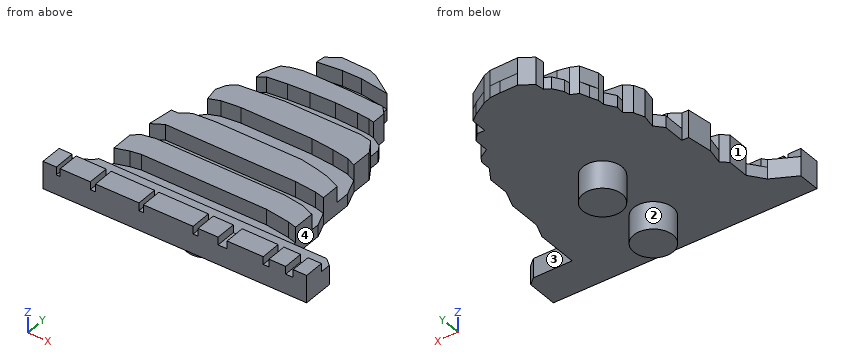
from build123d import *

# Parameters (mm, degrees)
F2_DEPTH  = 0.762
F4_DEPTH  = 1.016
F6_DEPTH  = 1.016
F8_DEPTH  = 0.5258
F0_R      = 12.7
F10_DEPTH = 0.50448
F11_R     = 1.2664455111
F11_R_2   = 1.2714517288
F12_DEPTH = 1.778


with BuildPart() as f2:
    # F1 (on face) → F2 (new body)
    with BuildSketch(Plane.XY):
        Polygon((-8.301156573, -6.202286575), (-8.301156573, -7.6132696122), (8.7365023792, -7.5040537175), (8.7365023792, -5.5138876204), (8.2679493353, -5.1142387092), (5.7544014417, -5.1142387092), (5.7544014417, -2.8919042088), (5.7544014417, -2.4577556178), (5.3745214827, -1.4809214044), (5.3745214827, -0.9925042978), (5.3745214827, 0), (5.3745214827, 0.6355526857), (4.9403728917, 1.7751924461), (4.9403728917, 2.4806838483), (4.9403728917, 3.1319067348), (4.3976870365, 4.000203684), (4.3976870365, 4.6514268033), (4.1806129739, 5.0313062966), (3.529390553, 5.4111862555), (3.529390553, 6.3337520696), (3.0952417292, 6.8221688271), (2.6068247389, 6.8221688271), (2.6068247389, 7.853272371), (2.1184075158, 8.2331513986), (1.1958420509, 8.7758377194), (0.6879131543, 8.9615155011), (0, 9.0042492375), (-1.1481875752, 9.0042492375), (-1.9346952904, 8.4792003036), (-2.0060034003, 7.9075405374), (-2.3858833592, 7.6904660091), (-2.7657633182, 7.0935124531), (-2.8200319503, 6.7136320285), (-3.3084489405, 6.4965579659), (-3.5255230032, 5.8996034786), (-3.7425975315, 5.4111862555), (-3.7425975315, 4.9770376645), (-4.1767461225, 4.3258150108), (-4.1224774905, 3.8373982534), (-4.5566260815, 3.4575182945), (-4.8279687762, 2.8062951751), (-4.6651633456, 1.9379982259), (-5.1535801031, 1.3953124871), (-5.1535801031, 0), (-5.5877286941, 0), (-5.8048027568, -1.6437270679), (-5.5877286941, -2.6748299133), (-6.0218772851, -3.0547098722), (-6.0218772851, -4.4656926766), (-6.7273690365, -5.3882584907), align=None)
    extrude(amount=F2_DEPTH)

    # F3 (on face) → F4 (join)
    with BuildSketch(Plane.XY.offset(0.762)):
        Polygon((-8.301156573, -7.6132696122), (8.7365023792, -7.5040537175), (8.7365023792, -5.5138876204), (8.2679493353, -5.1142387092), (5.7544014417, -5.1142387092), (-6.5178244245, -5.1142387092), (-6.7273690365, -5.3882584907), (-8.301156573, -6.202286575), align=None)
    extrude(amount=F4_DEPTH)

    # F5 (on face) → F6 (join)
    with BuildSketch(Plane.XY.offset(0.762)):
        Polygon((-1.9346952904, 8.4792003036), (-2.0060034003, 7.9075405374), (-0.4768302024, 8.0958995968), (0.7676923415, 8.1118550152), (2.6068247389, 7.853272371), (1.1958420509, 8.7758377194), (0.6879131543, 8.9615155011), (-1.1481875752, 9.0042492375), align=None)
        Polygon((-2.1202382632, 6.8673328497), (-2.8200319503, 6.7136320285), (-3.3084489405, 6.4965579659), (-3.7425975315, 5.4111862555), (-3.7425975315, 4.9770376645), (-3.3328498248, 5.2877464332), (-2.0883274265, 5.4473006167), (-0.7002060302, 5.5430331267), (0.927246525, 5.6068548001), (2.3791892454, 5.5589885451), (3.1769601628, 5.4951668717), (3.529390553, 5.4111862555), (3.529390553, 6.3337520696), (3.0952417292, 6.8221688271), (2.6068247389, 6.8221688271), (0.9432018269, 6.8992436863), (-1.290556509, 6.8992436863), align=None)
        Polygon((-2.7597796666, 3.9888094114), (-4.1224774905, 3.8373982534), (-4.5566260815, 3.4575182945), (-4.8279687762, 2.8062951751), (-4.6651633456, 1.9379982259), (-4.0006320924, 2.1927114576), (-2.8066006489, 2.334858058), (-1.3140613446, 2.334858058), (0.1642632997, 2.334858058), (1.7989494372, 2.334858058), (3.263059305, 2.2069262341), (4.3575884774, 2.0363503136), (4.9403728917, 1.7751924461), (4.9403728917, 3.1319067348), (4.3976870365, 4.000203684), (3.6326404661, 4.1401199996), (2.3959649261, 4.1401199996), (0.8465670398, 4.1401199996), (-1.2998466846, 4.1401199996), align=None)
        Polygon((-5.5877286941, 0), (-5.8048027568, -1.6437270679), (-5.076691974, -1.2083072215), (-3.9773182943, -1.2083072215), (-1.5074934345, -1.2083072215), (0.9020918515, -1.2083072215), (3.3719167113, -1.2083072215), (4.7423685901, -1.3287864858), (5.3745214827, -1.4809214044), (5.3745214827, -0.2745929523), (4.4110501185, 0.1470844581), (3.5074558109, 0.3579231852), (2.4683221709, 0.5386420526), (0, 0.5386420526), (-3.1490232795, 0.5386420526), (-4.53453511, 0.4181628174), (-5.1535801031, 0), align=None)
        Polygon((-5.5877286941, -2.6748299133), (-6.0218772851, -3.0547098722), (-6.0218772851, -4.4656926766), (-5.1821111701, -4.1901692748), (-4.5194751583, -4.0696901269), (-2.0044704434, -4.0696901269), (1.4593084343, -4.0696901269), (3.5978152882, -4.0696901269), (5.1791053265, -4.2805285193), (5.7544014417, -4.4461875223), (5.7544014417, -3.0154963024), (4.9230875447, -2.6841785293), (3.5978152882, -2.4995030768), (1.3388292864, -2.4995030768), (-2.4412076455, -2.4995030768), (-4.7549253743, -2.4995030768), align=None)
    extrude(amount=F6_DEPTH)

    # F7 (on face) → F8 (cut)
    with BuildSketch(Plane.XY.offset(1.778)):
        Polygon((-6.7273690365, -5.3882584907), (-8.301156573, -6.202286575), (8.7365023792, -6.202286575), (8.7365023792, -5.5138876204), (8.2679493353, -5.1142387092), (-6.5178244245, -5.1142387092), align=None)
    extrude(amount=-F8_DEPTH, mode=Mode.SUBTRACT)

    # F9 (on face) + F0 (on Top) → F10 (cut)
    with BuildSketch(Plane.XY.offset(1.778)):
        Polygon((-7.4496113843, -6.202286575), (-7.4406019717, -7.6077532299), (-7.1891224943, -7.60614118), (-7.1891224943, -6.202286575), align=None)
        Polygon((-5.2457139827, -6.202286575), (-5.2457139827, -7.593683418), (-4.905404364, -7.5915019435), (-4.9143096015, -6.202286575), align=None)
        Polygon((-2.0974383224, -6.202286575), (-2.0974383224, -7.5735021394), (-1.8112884347, -7.571667843), (-1.8200665304, -6.202286575), align=None)
        Polygon((7.377400318, -6.202286575), (7.3858004916, -7.5127120734), (7.8655239195, -7.5096369195), (7.8655239195, -6.202286575), align=None)
        Polygon((5.9232353463, -6.202286575), (5.9316952713, -7.522033272), (6.3001448289, -7.519671413), (6.3001448289, -6.202286575), align=None)
        Polygon((3.014677437, -6.202286575), (3.014677437, -7.5407321269), (3.5971800525, -7.5369981313), (3.5886241988, -6.202286575), align=None)
        Polygon((1.3927921775, -6.202286575), (1.4014382575, -7.5510734162), (1.7183985864, -7.5490416168), (1.7097655308, -6.202286575), align=None)
    with BuildSketch(Plane.XY):
        Circle(F0_R)
    extrude(amount=-F10_DEPTH, mode=Mode.SUBTRACT)

    # F11 (on face) → F12 (join)
    with BuildSketch(Plane.XY):
        Circle(F11_R)
        with Locations((0, -4.4713900425)):
            Circle(F11_R_2)
    extrude(amount=-F12_DEPTH)


solid = f2.part
The model under review builds one solid part; all positions refer to its coordinate system, in mm. Face numbers are marked on the shaded views. A direction names the side the tool comes from. Round coordinates to 2 decimals unless told otherwise and drop trailing zeros. Order: outer loops, then holes, each group sorted by start corner. A loop starts at its lowest first (then second) coordinate and runs counter-clockwise, first axis right, second up. Notation, with made-up numbers: (48.5, 75.5) -> (81.5, 75.5) arc R10 cw to (81.5, 93.5) -> close; hole circle Ø11 at (-17, -22.5). An arc over 180 degrees is marked (long way). Use CSV: the item, a comma, the result in double quotes. Start each with the question number.
(1) Insertion check: pin 1 (0.5 mm diameter, centred on y = -4, z = 1, fed in from +X); pin 2 (1.5 mm diameter, centred on x = -0.5, y = 6, fed in from -Z); pin 3 (1.5 mm diameter, centred on x = -4, z = -1.5, fed in from +Y); pin 4 (1.5 mm diameter, centred on y = 7, z = 0, fed in from +X). Each pin has a flat end and moves straight along its axis. Give the tip position at first contact, or say it passes through.
(2) Tool access review of the marked faces 1, 2, 3 and 4: name each direction out of +Z, -Z, +X, -X, +Y, -Y from which nothing blocks a thin tool from reaching the whole face with its end or side.
(3) Consider section B-B on y = -1. Write out the cut boundary in (x, z), and give its area (3 significant figures).
(4) Consider section A-A on z = -0.85. Write out the cut boundary in (x, y).
(5) Wall thickness on probe 1 along Y at (x, z) = (-3.25, 1.6); probe 2 along Y at (x, z) = (-5, 0.9); probe 3 along Y at (x, z) = (1, -0.75): over which ranges is each line inside the solid? List them lowest first. Write a range as from..to.
(6) Consider section C-C on x = 7. Write out the cut boundary in (y, z), and give its area (3 significant figures).
Responses:
1,pin 1,"x = 5.75"
1,pin 2,"z = 0"
1,pin 3,"through"
1,pin 4,"x = 3.53"
2,face 1,"+Z, -Z, -X, +Y"
2,face 2,"-Z"
2,face 3,"+Z, +X"
2,face 4,"+Z, -Z, +X, +Y"
3,outline,"(-5.72, 0) -> (-0.78, 0) -> (-0.78, -1.78) -> (0.78, -1.78) -> (0.78, 0) -> (5.37, 0) -> (5.37, 1.78) -> (-5.72, 1.78) -> close"
3,area,"22.5 mm²"
4,outline,"circle Ø2.54 at (0, -4.47); circle Ø2.53 at (0, 0)"
5,probe 1,"-7.58..-6.2, -4.07..-2.5, -1.21..0.53, 2.28..3.93, 5.3..6.52"
5,probe 2,"-7.59..-5.11, -4.16..-2.55, -1.21..0.1"
5,probe 3,"-5.26..-3.69, -0.78..0.78"
6,outline,"(-7.52, 0) -> (-5.11, 0) -> (-5.11, 1.25) -> (-6.2, 1.25) -> (-6.2, 1.78) -> (-7.52, 1.78) -> close"
6,area,"3.70 mm²"
